Source: CAD feature listing. Evaluate the final solid. Frame: model axes, mm. Face numbers are marked on the shaded views. A direction names the side the tool comes from. Give positions to 0.01 mm unless a question says otherwise; leave off trailing zeros. Order: outer loops, then holes, each group sorted by start corner. A loop starts at its lowest first (then second) coordinate and runs counter-clockwise, first axis right, second up. Notation, with made-up numbers: (26, 77.25) -> (84, 77.25) arc R15 cw to (84, 85.25) -> close; hole circle Ø1 at (43, 29.25). An arc over 180 degrees is marked (long way). Use CSV: the item, a comma, the result in double quotes.
```python
from build123d import *

# Parameters (mm, degrees)
SKETCH_2_R               = 22
EXTRUDE_1_DEPTH          = 10
SKETCH_3_R               = 20
CUT_EXTRUDE_1_DEPTH      = 4
CUT_EXTRUDE_START        = -3
SKETCH_4_R               = 22
SKETCH_4_R_2             = 12.7
CUT_EXTRUDE_2_DEPTH      = 3
SKETCH_9_R               = 20.15
CUT_EXTRUDE_3_DEPTH      = 4
CUT_EXTRUDE_START_2      = -0.5
SKETCH_10_R              = 22
SKETCH_10_R_2            = 15
CUT_EXTRUDE_4_DEPTH      = 0.5
PATTERN_CIRCULAR_1_COUNT = 4


with BuildPart() as part:
    # 草图2 → 凸台-拉伸1 (new body)
    with BuildSketch(Plane(origin=(0, 0, 0), x_dir=(1, 0, 0), z_dir=(0, 1, 0))):
        with Locations(Location((0, 0, 0), (0, 0, 270))):
            Circle(SKETCH_2_R)
    extrude(amount=EXTRUDE_1_DEPTH)

    # 草图3 → 切除-拉伸1 (cut)
    with BuildSketch(Plane.XZ):
        with Locations(Location((0, 0, 0), (0, 0, 270))):
            Circle(SKETCH_3_R)
    extrude(amount=-CUT_EXTRUDE_1_DEPTH, mode=Mode.SUBTRACT)

    # 草图4 → 切除-拉伸2 (cut)
    with BuildSketch(Plane(origin=(0, 10, 0), x_dir=(1, 0, 0), z_dir=(0, 1, 0)).offset(CUT_EXTRUDE_START)):
        with Locations(Location((0, 0, 0), (0, 0, 270))):
            Circle(SKETCH_4_R)
        with Locations(Location((0, 0, 0), (0, 0, 270))):
            Circle(SKETCH_4_R_2, mode=Mode.SUBTRACT)
    extrude(amount=CUT_EXTRUDE_2_DEPTH, mode=Mode.SUBTRACT)

    # 草图9 → 切除-拉伸3 (cut)
    with BuildSketch(Plane.XZ):
        with Locations(Location((0, 0, 0), (0, 0, 270))):
            Circle(SKETCH_9_R)
    extrude(amount=-CUT_EXTRUDE_3_DEPTH, mode=Mode.SUBTRACT)

    # 草图10 → 切除-拉伸4 (cut)
    with BuildSketch(Plane(origin=(0, 7, 0), x_dir=(1, 0, 0), z_dir=(0, 1, 0)).offset(CUT_EXTRUDE_START_2)):
        with Locations(Location((0, 0, 0), (0, 0, 270))):
            Circle(SKETCH_10_R)
        with Locations(Location((0, 0, 0), (0, 0, 270))):
            Circle(SKETCH_10_R_2, mode=Mode.SUBTRACT)
    extrude(amount=CUT_EXTRUDE_4_DEPTH, mode=Mode.SUBTRACT)

    # 草图7 → #2-56 螺纹孔1 (revolve, cut)
    with BuildSketch(Plane(origin=(0, 2, -22), x_dir=(0, 1, 0), z_dir=(1, 0, 0))):
        Polygon((0, 0), (0, 5.53416509), (0.889, 5), (0.889, 0), align=None)
    hole_wizard_2_56_1 = revolve(axis=Axis((0, 2, -28.35), (0, 0, 1)), mode=Mode.SUBTRACT)

    # 阵列(圆周)1: #2-56 螺纹孔1 ×4 about axis
    pattern_circular_1_axis = Axis((0, 0, 0), (0, 1, 0))
    for i in range(1, PATTERN_CIRCULAR_1_COUNT):
        add(hole_wizard_2_56_1.rotate(pattern_circular_1_axis, i * 360 / PATTERN_CIRCULAR_1_COUNT), mode=Mode.SUBTRACT)


solid = part.part
```
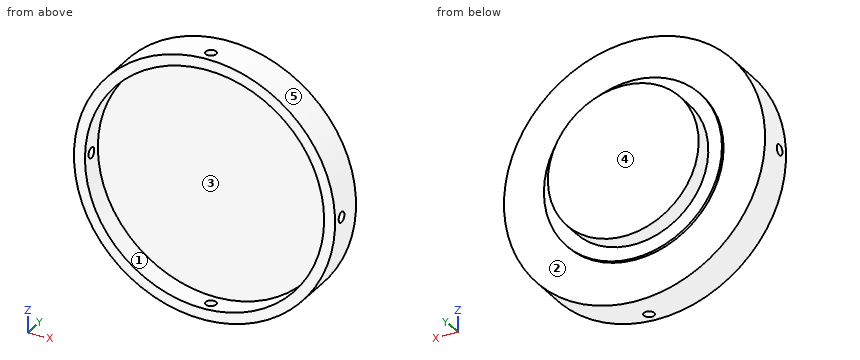
1. Section query D-D on z = 7. Return loops of the section in (x, y), plus the area to 3 significant figures.
Answer below:
outline,"(-20.86, 0) -> (-18.9, 0) -> (-18.9, 4) -> (18.9, 4) -> (18.9, 0) -> (20.86, 0) -> (20.86, 6.5) -> (13.27, 6.5) -> (13.27, 7) -> (10.6, 7) -> (10.6, 10) -> (-10.6, 10) -> (-10.6, 7) -> (-13.27, 7) -> (-13.27, 6.5) -> (-20.86, 6.5) -> close"
area,"197 mm²"
2. Mould query, pull axis Z, two halves, no side actions, for the marked faces 3, 4 and 5. Classes: released by +Z, released by -Z, zero draft, split by the parting line, or undercut.
Answer below:
face 3,"undercut"
face 4,"zero draft"
face 5,"split by the parting line"
3. Ray query, line 1 along Y through (x, z) = (-7.5, 11); line 2 along X through (y, z) = (0.75, -3); line 3 along Y through (x, z) = (-0.5, 17.5). Return the intervals inside material, ascending.
Answer below:
line 1,"y = 4 to 7"
line 2,"x = -21.79 to -19.93, 19.93 to 21.79"
line 3,"y = 4 to 6.5"
4. Section query B-B on z = 0. Return loops of the section in (x, y).
Answer below:
outline,"(-22, 0) -> (-20.15, 0) -> (-20.15, 1.11) -> (-22, 1.11) -> close; (-22, 2.89) -> (-20.15, 2.89) -> (-20.15, 4) -> (20.15, 4) -> (20.15, 2.89) -> (22, 2.89) -> (22, 6.5) -> (15, 6.5) -> (15, 7) -> (12.7, 7) -> (12.7, 10) -> (-12.7, 10) -> (-12.7, 7) -> (-15, 7) -> (-15, 6.5) -> (-22, 6.5) -> close; (20.15, 0) -> (22, 0) -> (22, 1.11) -> (20.15, 1.11) -> close"
5. Section query A-A on x = 0. Return loops of the section in (y, z), plus the area to 3 significant figures.
Answer below:
outline,"(0, -22) -> (1.11, -22) -> (1.11, -20.15) -> (0, -20.15) -> close; (0, 20.15) -> (1.11, 20.15) -> (1.11, 22) -> (0, 22) -> close; (2.89, -22) -> (6.5, -22) -> (6.5, -15) -> (7, -15) -> (7, -12.7) -> (10, -12.7) -> (10, 12.7) -> (7, 12.7) -> (7, 15) -> (6.5, 15) -> (6.5, 22) -> (2.89, 22) -> (2.89, 20.15) -> (4, 20.15) -> (4, -20.15) -> (2.89, -20.15) -> close"
area,"209 mm²"
6. Section query C-C on y = 2. Return loops of the section in (x, z), plus the area to 3 significant figures.
Answer below:
outline,"(-21.98, -0.89) arc R22 ccw to (-0.89, -21.98) -> (-0.89, -20.13) arc R20.15 cw to (-20.13, -0.89) -> close; (-21.98, 0.89) -> (-20.13, 0.89) arc R20.15 cw to (-0.89, 20.13) -> (-0.89, 21.98) arc R22 ccw to start; (0.89, -21.98) arc R22 ccw to (21.98, -0.89) -> (20.13, -0.89) arc R20.15 cw to (0.89, -20.13) -> close; (0.89, 20.13) arc R20.15 cw to (20.13, 0.89) -> (21.98, 0.89) arc R22 ccw to (0.89, 21.98) -> close"
area,"232 mm²"
7. Pin query (flat end, axial travel): P1, Ø8, axis at x = -2.5, z = -2.5, coming from the -Y side; P2, Ø5, axis at y = 6.5, z = 3.5, coming from the +X side; P3, Ø1.5, axis at y = 5.5, z = -2.5, coming from the -X side. Return the tip coordinate at first contact, or that it passes through.
Answer below:
P1,"stops at y = 4"
P2,"stops at x = 21.98"
P3,"stops at x = -21.93"
8. Access query for the marked faces 1 and 2. Directions: +Z, -Z, +X, -X, +Y, -Y. A direction counts if a zero-diameter tool reaches every point of the face in a straight line with its end or side. Return the directions, or none.
Answer below:
face 1,"-Y"
face 2,"+Y"
